from build123d import *

# Parameters (mm, degrees)
SKETCH1_W           = 300
SKETCH1_H           = 300
BOSS_EXTRUDE1_DEPTH = 150


# Read off the part's stored shape, not the designer's step: Cavity1
with BuildPart() as part:
    # Sketch1 → Boss-Extrude1 (new body)
    with BuildSketch(Plane(origin=(0, 0, 0), x_dir=(1, 0, 0), z_dir=(0, 1, 0))):
        Rectangle(SKETCH1_W, SKETCH1_H)
    extrude(amount=BOSS_EXTRUDE1_DEPTH)

    # Cavity1 outline → Cavity1 (revolve, cut)
    with BuildSketch(Plane(origin=(0, 152.053618149, 0), x_dir=(0, 1, 0), z_dir=(0, 0, -1))):
        with BuildLine():
            Line((41.5, 61.660319704), (2.053618149, 61.660319704))
            Line((2.053618149, 61.660319704), (2.053618149, -44.379680296))
            Line((2.053618149, -44.379680296), (41.5, -44.379680296))
            ThreePointArc((41.5, -44.379680296), (41.712132035, -44.291812331), (41.8, -44.079680296))
            Line((41.8, -44.079680296), (41.8, -30.439680296))
            ThreePointArc((41.8, -30.439680296), (41.712132034, -30.227548262), (41.5, -30.139680296))
            Line((41.5, -30.139680296), (22, -30.139680296))
            ThreePointArc((22, -30.139680296), (21.787867965, -30.051812331), (21.7, -29.839680296))
            Line((21.7, -29.839680296), (21.7, 47.120319704))
            ThreePointArc((21.7, 47.120319704), (21.787867966, 47.332451738), (22, 47.420319704))
            Line((22, 47.420319704), (41.5, 47.420319704))
            ThreePointArc((41.5, 47.420319704), (41.712132035, 47.508187669), (41.8, 47.720319704))
            Line((41.8, 47.720319704), (41.8, 61.360319704))
            ThreePointArc((41.8, 61.360319704), (41.712132034, 61.572451738), (41.5, 61.660319704))
        make_face()
    revolve(axis=Axis((0, 152.053618149, 0), (1, 0, 0)), mode=Mode.SUBTRACT)


solid = part.part
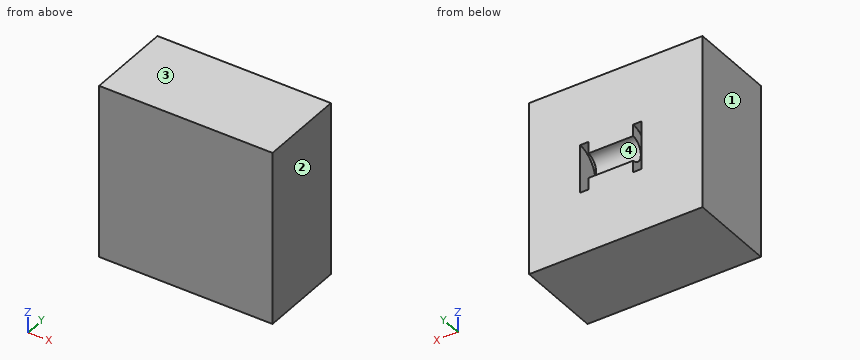
Work out the finished part from the listing and answer in its coordinate system (mm). Face numbers are marked on the shaded views. Give positions to 0.01 mm unless a question says otherwise; leave off trailing zeros. Write each loop counter-clockwise with the first axis right and the second up, starting at its lowest first coordinate (ties: lowest second). Pieces come first, ordered by that corner, then holes.
Q1. Straight lines are drawn through the part: L1, parallel to Z at x = 9.5, y = 138; L2, parallel to Y at x = 17, z = -13.5; L3, parallel to Y at x = 14.5, z = 15. For each, find the intervals that lie inside material, in ascending order.
Answer:
L1: z = -150 to -16.53, 16.53 to 150
L2: y = 0 to 135.06
L3: y = 0 to 136.37
Q2. The part is cut by section B-B on y = 123. State how many separate pieces and enclosed holes the cut face has, and give its area (3 significant figures).
Answer:
separate pieces: 1
enclosed holes: 2
area: 88,300 mm2
Q3. For a pull along X with two mould halves and no side action, classify the marked faces 1, 2, 3 and 4 as released by +X, released by -X, zero draft, split by the parting line, or undercut.
Answer:
face 1: released by -X
face 2: released by +X
face 3: zero draft
face 4: undercut
Q4. The part is cut by section A-A on z = 0. Give the vertices of the cut face in (x, y), and give its area (3 significant figures).
Answer:
outline: (-150, 0) - (150, 0) - (150, 150) - (61.66, 150) - (61.66, 110.55) arc R0.3 cw to (61.36, 110.25) - (47.72, 110.25) arc R0.3 cw to (47.42, 110.55) - (47.42, 130.05) arc R0.3 ccw to (47.12, 130.35) - (-29.84, 130.35) arc R0.3 ccw to (-30.14, 130.05) - (-30.14, 110.55) arc R0.3 cw to (-30.44, 110.25) - (-44.08, 110.25) arc R0.3 cw to (-44.38, 110.55) - (-44.38, 150) - (-150, 150) - close
area: 42,300 mm2
